Verification items for the finished model (mm, model axes). Round coordinates to 2 decimals unless told otherwise and drop trailing zeros. One line per item, written item: value.
from build123d import *

# Parameters (mm, degrees)
SKETCH_1_W          = 123
SKETCH_1_H          = 35
EXTRUDE_1_DEPTH     = 3
SKETCH_2_R          = 0.6
CUT_EXTRUDE_1_DEPTH = 65.011717677
SKETCH_2_3_R        = 1
CUT_EXTRUDE_2_DEPTH = 1.5
SKETCH_3_W          = 3
SKETCH_3_H          = 3
CUT_EXTRUDE_3_DEPTH = 2


with BuildPart() as part:
    # Sketch 1 → Extrude 1 (new body)
    with BuildSketch(Plane(origin=(0, 0, 0), x_dir=(1, 0, 0), z_dir=(0, 1, 0))):
        Rectangle(SKETCH_1_W, SKETCH_1_H)
    extrude(amount=EXTRUDE_1_DEPTH)

    # Sketch 2 → Cut-Extrude 1 (cut, through all)
    with BuildSketch(Plane.XZ):
        with Locations(Location((-30.75, 16, 0), (0, 0, 270))):
            Circle(SKETCH_2_R)
        with Locations(Location((30.75, 16, 0), (0, 0, 270))):
            Circle(SKETCH_2_R)
        with Locations(Location((-30.75, -16, 0), (0, 0, 270))):
            Circle(SKETCH_2_R)
        with Locations(Location((30.75, -16, 0), (0, 0, 270))):
            Circle(SKETCH_2_R)
        with Locations(Location((0, 16, 0), (0, 0, 270))):
            Circle(SKETCH_2_R)
        with Locations(Location((0, -16, 0), (0, 0, 270))):
            Circle(SKETCH_2_R)
        with Locations(Location((60, 8.75, 0), (0, 0, 270))):
            Circle(SKETCH_2_R)
        with Locations(Location((60, -8.75, 0), (0, 0, 270))):
            Circle(SKETCH_2_R)
    extrude(amount=-CUT_EXTRUDE_1_DEPTH, mode=Mode.SUBTRACT)

    # Sketch 2_3 → Cut-Extrude 2 (cut)
    with BuildSketch(Plane.XZ):
        with Locations(Location((-30.75, 16, 0), (0, 0, 270))):
            Circle(SKETCH_2_3_R)
        with Locations(Location((30.75, 16, 0), (0, 0, 270))):
            Circle(SKETCH_2_3_R)
        with Locations(Location((-30.75, -16, 0), (0, 0, 270))):
            Circle(SKETCH_2_3_R)
        with Locations(Location((30.75, -16, 0), (0, 0, 270))):
            Circle(SKETCH_2_3_R)
        with Locations(Location((0, 16, 0), (0, 0, 270))):
            Circle(SKETCH_2_3_R)
        with Locations(Location((0, -16, 0), (0, 0, 270))):
            Circle(SKETCH_2_3_R)
        with Locations(Location((60, 8.75, 0), (0, 0, 270))):
            Circle(SKETCH_2_3_R)
        with Locations(Location((60, -8.75, 0), (0, 0, 270))):
            Circle(SKETCH_2_3_R)
    extrude(amount=-CUT_EXTRUDE_2_DEPTH, mode=Mode.SUBTRACT)

    # Sketch 3 → Cut-Extrude 3 (cut)
    with BuildSketch(Plane.XZ):
        with Locations((58.5, -14.5)):
            Rectangle(SKETCH_3_W, SKETCH_3_H)
        with Locations((58.5, 14.5)):
            Rectangle(SKETCH_3_W, SKETCH_3_H)
        with Locations((58.5, 0)):
            Rectangle(SKETCH_3_W, SKETCH_3_H)
        with Locations((36.9, 14.5)):
            Rectangle(SKETCH_3_W, SKETCH_3_H)
        with Locations((12.3, 14.5)):
            Rectangle(SKETCH_3_W, SKETCH_3_H)
        with Locations((-12.3, 14.5)):
            Rectangle(SKETCH_3_W, SKETCH_3_H)
        with Locations((-36.9, 14.5)):
            Rectangle(SKETCH_3_W, SKETCH_3_H)
        with Locations((36.9, -14.5)):
            Rectangle(SKETCH_3_W, SKETCH_3_H)
        with Locations((36.896881316, -95.946698649)):
            Rectangle(SKETCH_3_W, SKETCH_3_H)
        with Locations((12.3, -14.5)):
            Rectangle(SKETCH_3_W, SKETCH_3_H)
        with Locations((-12.3, -14.5)):
            Rectangle(SKETCH_3_W, SKETCH_3_H)
        with Locations((-36.9, -14.5)):
            Rectangle(SKETCH_3_W, SKETCH_3_H)
    extrude(amount=-CUT_EXTRUDE_3_DEPTH, mode=Mode.SUBTRACT)


solid = part.part
(1) Mould release check, pull along X, two halves, no side actions. Record for faces 1 (the face through (12, 2, -14)), 2 (the face through (61.5, 1, 0)), 3 (the face through (-1, 0, 0)): +X half, -X half, draft (parallel to the pull), parting line (faces both ways), or undercut.
Completed:
face 1: undercut
face 2: +X half
face 3: draft
(2) Thickness scan on L1, parallel to X at y = 2.75, z = -16; L2, parallel to X at y = 2.6, z = 16.5. Record the ranges inside material, lowest first. Write a range as from..to.
Completed:
L1: x = -61.5..-31.35, -30.15..-0.6, 0.6..30.15, 31.35..61.5
L2: x = -61.5..-31.08, -30.42..-0.33, 0.33..30.42, 31.08..61.5
(3) Depth check by flat-ended pin: pin 1 Ø1.6 at (x, z) = (0, 16) entering from -Y. Enter the tip coordinate at first touch or a pass-through.
Completed:
pin 1: stops at y = 1.5
